from build123d import *

# Parameters (mm, degrees)
F1_DEPTH = 152.4


with BuildPart() as f1:
    # F0 (on Front) → F1 (new body)
    with BuildSketch(Plane.XZ):
        with BuildLine():
            Line((-8.916182, 0), (0, 0))
            Line((0, 0), (0, 2.54))
            Line((0, 2.54), (-9.672946, 2.54))
            Line((-9.672946, 2.54), (-3.850629, 35.56))
            Line((-3.850629, 35.56), (50.007153, 35.56))
            ThreePointArc((50.007153, 35.56), (53.680685, 36.897056), (55.63533, 40.282601))
            Line((55.63533, 40.282601), (59.281313, 60.96))
            Line((59.281313, 60.96), (113.671924, 60.96))
            Line((113.671924, 60.96), (123.972946, 2.54))
            Line((123.972946, 2.54), (114.3, 2.54))
            Line((114.3, 2.54), (114.3, 0))
            Line((114.3, 0), (123.216182, 0))
            ThreePointArc((123.216182, 0), (125.648373, 1.134149), (126.342947, 3.726333))
            Line((126.342947, 3.726333), (116.26586, 60.876333))
            ThreePointArc((116.26586, 60.876333), (115.179946, 62.757191), (113.139095, 63.5))
            Line((113.139095, 63.5), (59.814141, 63.5))
            ThreePointArc((59.814141, 63.5), (57.773291, 62.757191), (56.687377, 60.876333))
            Line((56.687377, 60.876333), (53.133918, 40.723667))
            ThreePointArc((53.133918, 40.723667), (52.048004, 38.842809), (50.007153, 38.1))
            Line((50.007153, 38.1), (-3.317801, 38.1))
            ThreePointArc((-3.317801, 38.1), (-5.358651, 37.357191), (-6.444565, 35.476333))
            Line((-6.444565, 35.476333), (-12.042947, 3.726333))
            ThreePointArc((-12.042947, 3.726333), (-11.348373, 1.134149), (-8.916182, 0))
        make_face()
    extrude(amount=F1_DEPTH)


solid = f1.part
The listing builds one solid part. Answer for the finished solid, in the listing's coordinates (mm). A direction names the side the tool comes from. Coordinates: 2 decimals unless noted, no trailing zeros. Loops run counter-clockwise (first coordinate to the right, second up) from the corner with the lowest first, then second, coordinate; pieces in that order, holes last.
1) Determine the mould class of faces 1 (the face through (-5, -75, 0)), 2 (the face through (119, -75, 2.54)), 3 (the face through (-9.205, -75.133, 19.824)) for opening direction Z: pulls with the +Z half, pulls with the -Z half, needs draft (parallel to the pull), parting line crosses it, or undercut.
2) A tool of negligible diameter and unlimited length cuts with its end or side. For faces 4 (the face through (52, 0, 37)), 5 (the face through (86, -75, 60.96)), 6 (the face through (119, -75, 0)), 7 (the face through (24, -75, 38.1)), 8 (the face through (-6.803, -75.133, 18.819)), from which of +Z, -Z, +X, -X, +Y, -Y can it reach the whole face along a straight path? Write none if from no direction.
3) Flat-ended cylindrical pins translate along their axes: pin 1 Ø8 at (y, z) = (-26, 26.5) entering from -X; pin 2 Ø4 at (x, y) = (66, -98) entering from -Z; pin 3 Ø4 at (y, z) = (-124.5, 41) entering from +X. Find the tip coordinate at first contact, or state that the pin passes through.
4) Find the intervals of material crossed by L1, parallel to X at y = -36.5, z = 61; L2, parallel to X at y = -65, z = 13; L3, parallel to Z at x = 70, y = -48, in increasing order.
5) Find section B-B on z = 25. Write down the section's boundary in (x, y).
6) Find section A-A on y = -84.5. Write down the section's boundary in (x, z) (3 decimals).
7) Find section C-C on x = 75.5. Write down the section's boundary in (y, z).
Values:
1. face 1: pulls with the -Z half
1. face 2: undercut
1. face 3: pulls with the +Z half
2. face 4: +Z, -Z, +X, -X, +Y
2. face 5: -Z, +Y, -Y
2. face 6: -Z, +X, -X, +Y, -Y
2. face 7: +Z, -X, +Y, -Y
2. face 8: +Y, -Y
3. pin 1: stops at x = -8.73
3. pin 2: stops at z = 60.96
3. pin 3: stops at x = 120.12
4. L1: x = 56.71 to 116.24
4. L2: x = -10.41 to -7.83, 122.13 to 124.71
4. L3: z = 60.96 to 63.5
5. outline: (-8.29, -152.4) - (-5.71, -152.4) - (-5.71, 0) - (-8.29, 0) - close; (120.01, -152.4) - (122.59, -152.4) - (122.59, 0) - (120.01, 0) - close
6. outline: (-12.043, 3.726) arc R3.175 ccw to (-8.916, 0) - (0, 0) - (0, 2.54) - (-9.673, 2.54) - (-3.851, 35.56) - (50.007, 35.56) arc R5.715 ccw to (55.635, 40.283) - (59.281, 60.96) - (113.672, 60.96) - (123.973, 2.54) - (114.3, 2.54) - (114.3, 0) - (123.216, 0) arc R3.175 ccw to (126.343, 3.726) - (116.266, 60.876) arc R3.175 ccw to (113.139, 63.5) - (59.814, 63.5) arc R3.175 ccw to (56.687, 60.876) - (53.134, 40.724) arc R3.175 cw to (50.007, 38.1) - (-3.318, 38.1) arc R3.175 ccw to (-6.445, 35.476) - close
7. outline: (-152.4, 60.96) - (0, 60.96) - (0, 63.5) - (-152.4, 63.5) - close
